Geometry check sheet. Reference: the model listing, model coordinates, mm. A direction names the side the tool comes from. Round coordinates to 2 decimals unless told otherwise and drop trailing zeros. Loops run counter-clockwise (first coordinate to the right, second up) from the corner with the lowest first, then second, coordinate; pieces in that order, holes last. Notation, with made-up numbers: M 1.5,-28 L 18.5,-28 A21 cw 18.5,-21 Z; hole C -26,20 d1. An arc over 180 degrees is marked long. Answer in a Markdown table with one row per item. Add a question column.
```python
from build123d import *

# Parameters (mm, degrees)
BOSS_EXTRUDE1_DEPTH = 60
CUT_EXTRUDE1_DEPTH  = 60
FILLET19_R          = 0.5
FILLET20_R          = 0.5
FILLET22_R          = 1


with BuildPart() as part:
    # Sketch1 → Boss-Extrude1 (new body)
    with BuildSketch(Plane.XY):
        Polygon((-2, 3), (-2, 23), (2, 23), (2, 3), (6, 3), (6, -3), (-6, -3), (-6, 3), align=None)
    extrude(amount=BOSS_EXTRUDE1_DEPTH)

    # Sketch2 → Cut-Extrude1 (cut)
    with BuildSketch(Plane.XY.offset(60)):
        with BuildLine():
            Line((-6, -3), (6, -3))
            Line((6, -3), (6, 3))
            Line((6, 3), (1.5, 3))
            Line((1.5, 3), (1.5, 0.5))
            Line((1.5, 0.5), (3, 0.5))
            ThreePointArc((3, 0.5), (4.5, -1), (3, -2.5))
            Line((3, -2.5), (-3, -2.5))
            ThreePointArc((-3, -2.5), (-4.5, -1), (-3, 0.5))
            Line((-3, 0.5), (-1.5, 0.5))
            Line((-1.5, 0.5), (-1.5, 3))
            Line((-1.5, 3), (-6, 3))
            Line((-6, 3), (-6, -3))
        make_face()
    extrude(amount=-CUT_EXTRUDE1_DEPTH, mode=Mode.SUBTRACT)

    # Fillet19
    fillet19_edges = [part.edges().sort_by_distance(p)[0] for p in [
        (-2, 3, 30),
    ]]
    fillet(fillet19_edges, radius=FILLET19_R - 0.0001)  # a hair under: the kernel refuses the full size

    # Fillet20
    fillet20_edges = [part.edges().sort_by_distance(p)[0] for p in [
        (2, 3, 30),
    ]]
    fillet(fillet20_edges, radius=FILLET20_R - 0.0001)  # a hair under: the kernel refuses the full size

    # Fillet22
    fillet22_edges = [part.edges().sort_by_distance(p)[0] for p in [
        (-2, 23, 30),
        (2, 23, 30),
    ]]
    fillet(fillet22_edges, radius=FILLET22_R)


solid = part.part
```
1) Cross-section at B-B, the plane y = 21.25. Record the boundary of the cut face in (x, z).
2) Go/stop test with flat-tipped pins: pin 1 (5 mm diameter, centred on y = 11.5, z = 36, fed in from -X); pin 2 (2 mm diameter, centred on y = 6, z = 24, fed in from +X); pin 3 (0.8 mm diameter, centred on y = 1.5, z = 31.5, fed in from +X). Record where each tip stops, or that it passes through.
3) Set-up check for faces 1 (the flat face through (2, 13, 30)), 2 (the flat face through (-2, 0.5, 30)), 3 (the flat face through (0, 23, 30)), 4 (the flat face through (2, 0.5, 30)), 5 (the flat face through (-2, 13, 30)): record each of +Z, -Z, +X, -X, +Y, -Y from which the full face is reachable in a straight line by a thin tool's end or side.
4) Thickness scan on L1, parallel to Y at x = -2.5, z = 23; L2, parallel to X at y = 16.25, z = 55; L3, parallel to X at y = 1, z = 10. Record the ranges inside material, lowest first. Write a range as [from, to].
5) Draft check along Y on faces 6 (the flat face through (0, -2.5, 30)), 7 (the flat face through (-1.5, 2, 30)), 8 (the flat face through (0, 10, 0)). Enter one of: +Y half, -Y half, draft (parallel to the pull), parting line (faces both ways), or undercut.
Worked answers:
| question | item | result |
|---|---|---|
| 1 | outline | M -2,0 L 2,0 L 2,60 L -2,60 Z |
| 2 | pin 1 | stops at x = -2 |
| 2 | pin 2 | stops at x = 2 |
| 2 | pin 3 | stops at x = 1.5 |
| 3 | face 1 | +Z, -Z, +X, +Y |
| 3 | face 2 | +Z, -Z, -X |
| 3 | face 3 | +Z, -Z, +X, -X, +Y |
| 3 | face 4 | +Z, -Z, +X |
| 3 | face 5 | +Z, -Z, -X, +Y |
| 4 | L1 | y = [-2.5, 0.5] |
| 4 | L2 | x = [-2, 2] |
| 4 | L3 | x = [-1.5, 1.5] |
| 5 | face 6 | -Y half |
| 5 | face 7 | undercut |
| 5 | face 8 | draft |
